Autodesk Inventor part; units mm, degrees
ref_plane "YZ Plane" through (0, 0, 0) normal (1, 0, 0) x (0, 1, 0)
ref_plane "XZ Plane" through (0, 0, 0) normal (0, 1, 0) x (-1, 0, 0)
ref_plane "XY Plane" through (0, 0, 0) normal (0, 0, 1) x (1, 0, 0)
sketch "Sketch1" plane through (0, 0, 0) normal (0, 1, 0) x (-1, 0, 0)
  line L0 (120, -200) -> (-120, -200)
  line L1 (-120, -200) -> (-120, 200)
  line L2 (-120, 200) -> (120, 200)
  line L3 (120, 200) -> (120, -200)
  line L4 (120, -200) -> (-120, 200) construction
  line L5 (-120, -200) -> (120, 200) construction
  point P0 (0, 0)
  point P1 (0, 0)
  dimension "d16" = 240
  dimension "d17" = 400
extrude "Plate1" add sketch "Sketch1" along normal blind 8
sketch "Sketch2" plane through (0, 0, 0) normal (0, -1, 0) x (1, 0, 0)
  line L0 (100, 180) -> (100, -180) construction
  line L1 (-120, -200) -> (120, -200)
  line L2 (120, -200) -> (120, 200)
  line L3 (120, 200) -> (-120, 200)
  line L4 (-120, 200) -> (-120, -200)
  point P0 (100, 0)
  point P1 (100, 0)
  point P2 (0, 0)
  point P3 (100, 120)
  point P4 (100, -120)
  dimension "d19" = 20
  dimension "d20" = 20
  dimension "d21" = 360
  dimension "d22" = 120
  dimension "d23" = 120
hole "Hole1" at (100, 0, 180) at (100, 0, -180) at (100, 0, -120) at (100, 0, 120) direction (0, 1, 0) diameter 20 end through all
mirror "Mirror1" about plane through (0, 0, 0) normal (1, 0, 0) of "Hole1"
equation "\"d20\" = d19"
equation "\"d3\" = d19"
equation "\"d8\" = Thickness"
equation "\"d2\" = Thickness"
equation "\"BendRadius\" = Thickness"
equation "\"BendReliefWidth\" = Thickness"
equation "\"BendReliefDepth\" = 0.5 * Thickness"
equation "\"CornerReliefSize\" = 4 * Thickness"
equation "\"MinimumRemnant\" = 2 * Thickness"
equation "\"TransitionRadius\" = BendRadius"
equation "\"JacobiRadiusSize\" = BendRadius"
equation "\"GapSize\" = Thickness"
properties part number "Ухо на швеллер пямое"
Part model, mm, in its own coordinate system. Coordinates: 2 decimals unless noted, no trailing zeros. Loops run counter-clockwise (first coordinate to the right, second up) from the corner with the lowest first, then second, coordinate; pieces in that order, holes last. Notation, with made-up numbers: (-24, 24) - (30, 24) arc R22 ccw to (30, 47) - close; hole circle Ø5 at (0.25, 45.5). An arc over 180 degrees is marked (long way). Write each question's results on one line, items separated by ' | '. Start each with the question number.
Q1. Two-plate mould, pull along Z, no slides. Class faces 1 (the flat face through (2, 0, 3)), 2 (the cylindrical face through (-109.915, 4.056, -118.698)), 3 (the flat face through (2, 4, 200)), 4 (the flat face through (-2, 4, -200)): +Z half, -Z half, draft (parallel to the pull), parting line (faces both ways), or undercut.
Q2. Probe line 1 along Z through (x, y) = (-100, 2); line 2 along X through (y, z) = (1.75, -120); line 3 along Z through (x, y) = (-93, 6). List the from-to ranges inside material, lowest first.
Q3. Slice it at A-A on x = -100. Give the cut face in (y, z), and give its area (3 significant figures).
Q4. Slice it at B-B on z = 180. Give the cut face in (x, y).
Q5. Slice it at C-C on y = 6.5. Give the number of separate pieces and of enclosed holes in the cut face, and give its area (3 significant figures).
Answer:
1) face 1: draft | face 2: undercut | face 3: +Z half | face 4: -Z half
2) line 1: z = -200 to -190, -170 to -130, -110 to 110, 130 to 170, 190 to 200 | line 2: x = -120 to -110, -90 to 90, 110 to 120 | line 3: z = -200 to -187.14, -172.86 to -127.14, -112.86 to 112.86, 127.14 to 172.86, 187.14 to 200
3) outline: (0, -200) - (8, -200) - (8, -190) - (0, -190) - close; (0, -170) - (8, -170) - (8, -130) - (0, -130) - close; (0, -110) - (8, -110) - (8, 110) - (0, 110) - close; (0, 130) - (8, 130) - (8, 170) - (0, 170) - close; (0, 190) - (8, 190) - (8, 200) - (0, 200) - close | area: 2,560 mm2
4) outline: (-120, 0) - (-110, 0) - (-110, 8) - (-120, 8) - close; (-90, 0) - (90, 0) - (90, 8) - (-90, 8) - close; (110, 0) - (120, 0) - (120, 8) - (110, 8) - close
5) separate pieces: 1 | enclosed holes: 8 | area: 93,500 mm2
